For this review, take the finished solid that the model builds, in its own axes (mm). Face numbers are marked on the shaded views. A direction names the side the tool comes from. Round coordinates to 2 decimals unless told otherwise and drop trailing zeros. Write each loop counter-clockwise with the first axis right and the second up, starting at its lowest first coordinate (ties: lowest second). Pieces come first, ordered by that corner, then holes. Notation, with made-up numbers: M 62.25,58.25 L 106.25,58.25 A14 ccw 106.25,75.25 Z; hole C -38.5,61.5 d5. An arc over 180 degrees is marked long. Use one line per item in the form item = value. Start each with the question number.
Item 1: For the marked faces 1, 2 and 3, list the 3-axis set-ups (+Z, -Z, +X, -X, +Y, -Y) from which the entire face can be reached by the end or side of a thin tool; tool diameter is ignored.
Item 2: Add section D-D (y = 2.75). State the section outline as (x, z) points.
Item 3: Add section B-B (y = 7). State the section outline as (x, z) points, and give its area (3 significant figures).
Item 4: Draft analysis for pull direction X (two halves, no side actions). For the marked faces 4, 5, 6 and 7, state which applies: released by +X, released by -X, zero draft, split by the parting line, or undercut.
Item 5: Add section A-A (x = -7.5). State the section outline as (y, z) points.
Item 6: Add section C-C (z = 13). State the section outline as (x, y) points.
Item 7: For line 1 (Y direction, x = -9.75, z = 38); line 2 (X direction, y = 9.25, z = 7.5); line 3 (X direction, y = 4.5, z = 45), list the stretches that pass through material, from the lowest coordinate up. Write a range as [from, to].
Item 8: For P1, Ø4, axis at x = -11.5, y = 3.5, coming from the -Z side, flat-tipped, find the tip position at first contact; note if it passes through.
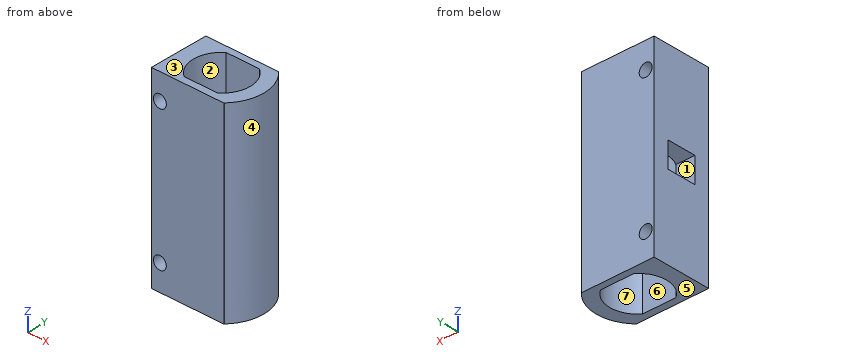
from build123d import *

# Parameters (mm, degrees)
SALIENTE_EXTRUIR1_DEPTH = 52
CROQUIS3_W              = 0.615681901
CROQUIS3_H              = 16
SALIENTE_EXTRUIR2_DEPTH = 52
CROQUIS2_R              = 1.75
CORTAR_EXTRUIR1_DEPTH   = 52
CROQUIS4_W              = 6.89100463
CROQUIS4_H              = 7.9059588
CORTAR_EXTRUIR2_DEPTH   = 10


with BuildPart() as part:
    # Croquis1 → Saliente-Extruir1 (new body)
    with BuildSketch(Plane.XY):
        with BuildLine():
            Line((-3.032251305, 15.708802589), (-22.152251305, 15.708802589))
            Line((-22.152251305, 15.708802589), (-22.152251305, -0.291197411))
            Line((-22.152251305, -0.291197411), (-3.132125677, -0.291197411))
            ThreePointArc((-3.132125677, -0.291197411), (-3.082032439, -0.241353267), (-3.032251305, -0.191197411))
            ThreePointArc((-3.032251305, -0.191197411), (0.228795467, 7.758802589), (-3.032251305, 15.708802589))
        make_face()
        with BuildLine():
            Line((-15.641976571, 13.908802589), (-6.542526038, 13.908802589))
            ThreePointArc((-6.542526038, 13.908802589), (-3.442251305, 7.758802589), (-6.542526038, 1.608802589))
            Line((-6.542526038, 1.608802589), (-15.641976571, 1.608802589))
            ThreePointArc((-15.641976571, 1.608802589), (-18.742251305, 7.758802589), (-15.641976571, 13.908802589))
        make_face(mode=Mode.SUBTRACT)
    extrude(amount=SALIENTE_EXTRUIR1_DEPTH)

    # Croquis3 → Saliente-Extruir2 (add)
    with BuildSketch(Plane.XY.offset(52)):
        with Locations((-22.460092256, 7.708802589)):
            Rectangle(CROQUIS3_W, CROQUIS3_H)
    extrude(amount=-SALIENTE_EXTRUIR2_DEPTH)

    # Croquis2 → Cortar-Extruir1 (cut)
    with BuildSketch(Plane(origin=(0, 15.708802589, 0), x_dir=(1, 0, 0), z_dir=(0, 1, 0))):
        with Locations(Location((-20.467933206, -7, 0), (0, 0, 270))):
            Circle(CROQUIS2_R)
        with Locations(Location((-20.467933206, -45, 0), (0, 0, 270))):
            Circle(CROQUIS2_R)
    extrude(amount=-CORTAR_EXTRUIR1_DEPTH, mode=Mode.SUBTRACT)

    # Croquis4 → Cortar-Extruir2 (cut)
    with BuildSketch(Plane.ZY.offset(22.767933206)):
        with Locations((26, 7.708802589)):
            Rectangle(CROQUIS4_W, CROQUIS4_H)
    extrude(amount=-CORTAR_EXTRUIR2_DEPTH, mode=Mode.SUBTRACT)


solid = part.part
Calculated:
q1.face_1 = -X
q1.face_2 = +Z, -Z
q1.face_3 = +Z, +X, -X, +Y, -Y
q2.outline = M -22.77,0 L -16.87,0 L -16.87,52 L -22.77,52 Z; M -5.31,0 L -0.94,0 L -0.94,52 L -5.31,52 Z; hole C -20.47,7 d3.5; hole C -20.47,45 d3.5
q3.outline = M -22.77,0 L -18.7,0 L -18.7,22.55 L -22.77,22.55 Z; M -22.77,29.45 L -18.7,29.45 L -18.7,52 L -22.77,52 Z; M -3.48,0 L 0.2,0 L 0.2,52 L -3.48,52 Z; hole C -20.47,7 d3.5; hole C -20.47,45 d3.5
q3.area = 356 mm^2
q4.face_4 = released by +X
q4.face_5 = zero draft
q4.face_6 = undercut
q4.face_7 = undercut
q5.outline = M -0.29,0 L 1.61,0 L 1.61,52 L -0.29,52 Z; M 13.91,0 L 15.71,0 L 15.71,52 L 13.91,52 Z
q6.outline = M -22.77,-0.29 L -3.13,-0.29 A11.32 ccw -3.03,-0.19 A11.32 ccw -3.03,15.71 L -22.77,15.71 Z; hole M -15.64,1.61 L -6.54,1.61 A7.65 ccw -6.54,13.91 L -15.64,13.91 A7.65 ccw Z
q7.line_1 = [-0.29, 1.61], [13.91, 15.71]
q7.line_2 = [-22.77, -22.14], [-18.79, -18.6], [-3.59, 0.13]
q7.line_3 = [-22.77, -22.22], [-18.72, -18.01], [-4.17, -0.25]
q8.P1 = 0
